from build123d import *

# Parameters (mm, degrees)
BOSS_EXTRUDE1_DEPTH  = 8.6
CHAMFER1_SIZE        = 1.414
CHAMFER1_EDGE_2_SIZE = 1.414
CHAMFER1_EDGE_3_SIZE = 1.414
CHAMFER1_EDGE_4_SIZE = 1.414
CHAMFER1_EDGE_5_SIZE = 1.414
CHAMFER1_EDGE_6_SIZE = 1.414
FILLET2_R            = 0.25
SKETCH6_R            = 1.5
CUT_EXTRUDE1_DEPTH   = 28
BOSS_EXTRUDE2_DEPTH  = 2.1
SKETCH9_R            = 2.75
CUT_EXTRUDE2_DEPTH   = 4.2
CHAMFER3_SIZE        = 0.75


with BuildPart() as part:
    # Sketch1 → Revolve1 (revolve)
    with BuildSketch(Plane.XY, mode=Mode.PRIVATE) as revolve1_sk:
        Polygon((0, 0), (6, 0), (6, 5.75), (4.875, 5.75), (4.875, 6.5), (7.75, 8), (7.75, 38.4), (8.7, 38.4), (8.7, 39.4), (0, 39.4), align=None)
    revolve(revolve1_sk.sketch.rotate(Axis((0, 39.4, 0), (0, -1, 0)), 180), axis=Axis((0, 39.4, 0), (0, -1, 0)))

    # Sketch3 → Boss-Extrude1 (add)
    with BuildSketch(Plane(origin=(0, 39.4, 0), x_dir=(1, 0, 0), z_dir=(0, 1, 0))):
        Polygon((0, 9.814954576), (-8.5, 4.907477288), (-8.5, -4.907477288), (0, -9.814954576), (8.5, -4.907477288), (8.5, 4.907477288), align=None)
    extrude(amount=BOSS_EXTRUDE1_DEPTH)

    # Chamfer1
    chamfer1_edges = [part.edges().sort_by_distance(p)[0] for p in [
        (8.5, 43.7, -4.907477288),
    ]]
    chamfer(chamfer1_edges, length=CHAMFER1_SIZE)

    # Chamfer1 edge 2
    chamfer1_edge_2_edges = [part.edges().sort_by_distance(p)[0] for p in [
        (0, 43.7, -9.814954576),
    ]]
    chamfer(chamfer1_edge_2_edges, length=CHAMFER1_EDGE_2_SIZE)

    # Chamfer1 edge 3
    chamfer1_edge_3_edges = [part.edges().sort_by_distance(p)[0] for p in [
        (-8.5, 43.7, -4.907477288),
    ]]
    chamfer(chamfer1_edge_3_edges, length=CHAMFER1_EDGE_3_SIZE)

    # Chamfer1 edge 4
    chamfer1_edge_4_edges = [part.edges().sort_by_distance(p)[0] for p in [
        (-8.5, 43.7, 4.907477288),
    ]]
    chamfer(chamfer1_edge_4_edges, length=CHAMFER1_EDGE_4_SIZE)

    # Chamfer1 edge 5
    chamfer1_edge_5_edges = [part.edges().sort_by_distance(p)[0] for p in [
        (0, 43.7, 9.814954576),
    ]]
    chamfer(chamfer1_edge_5_edges, length=CHAMFER1_EDGE_5_SIZE)

    # Chamfer1 edge 6
    chamfer1_edge_6_edges = [part.edges().sort_by_distance(p)[0] for p in [
        (8.5, 43.7, 4.907477288),
    ]]
    chamfer(chamfer1_edge_6_edges, length=CHAMFER1_EDGE_6_SIZE)

    # Sketch5 → Revolve2 (revolve)
    with BuildSketch(Plane.XY, mode=Mode.PRIVATE) as revolve2_sk:
        Polygon((7.75, 28.801965379), (10.5, 28.801965379), (10.5, 26.801965379), (8.7, 26.801965379), (8.7, 23.801965379), (7.75, 23.801965379), align=None)
    revolve(revolve2_sk.sketch.rotate(Axis((0, 0, 0), (0, 1, 0)), 180), axis=Axis((0, 0, 0), (0, 1, 0)))

    # Fillet2
    fillet2_edges = [part.edges().sort_by_distance(p)[0] for p in [
        (10.5, 28.801965379, 0),
        (10.5, 26.801965379, 0),
        (8.7, 23.801965379, 0),
    ]]
    fillet(fillet2_edges, radius=FILLET2_R)

    # Sketch6 → Cut-Extrude1 (cut)
    with BuildSketch(Plane.XZ):
        Circle(SKETCH6_R)
    extrude(amount=-CUT_EXTRUDE1_DEPTH, mode=Mode.SUBTRACT)

    # Sketch7 → Boss-Extrude2 (add, symmetric)
    with BuildSketch(Plane.XY):
        with BuildLine():
            Line((4.5, 54.25), (4.5, 48))
            Line((4.5, 48), (-4.5, 48))
            Line((-4.5, 48), (-4.5, 54.25))
            ThreePointArc((-4.5, 54.25), (0, 58.75), (4.5, 54.25))
        make_face()
    extrude(amount=BOSS_EXTRUDE2_DEPTH, both=True)

    # Sketch8 → Cut-Revolve1 (revolve, cut)
    with BuildSketch(Plane.XY):
        with BuildLine():
            Line((0, 57.15), (0, 51.35))
            ThreePointArc((0, 51.35), (2.9, 54.25), (0, 57.15))
        make_face()
    revolve(axis=Axis((0, 48, 0), (0, 1, 0)), mode=Mode.SUBTRACT)

    # Sketch10 → Cut-Revolve2 (revolve, cut)
    with BuildSketch(Plane.XY, mode=Mode.PRIVATE) as cut_revolve2_sk:
        Polygon((7, 48), (8.5, 46.6), (10.124681139, 45.083630937), (10.124681139, 47.819402207), (7, 50.73577127), align=None)
    revolve(cut_revolve2_sk.sketch.rotate(Axis((0, 0, 0), (0, 1, 0)), 90), axis=Axis((0, 0, 0), (0, 1, 0)), mode=Mode.SUBTRACT)

    # Sketch9 → Cut-Extrude2 (cut)
    with BuildSketch(Plane.XY.offset(2.1)):
        with Locations((0, 54.25)):
            Circle(SKETCH9_R)
    extrude(amount=-CUT_EXTRUDE2_DEPTH, mode=Mode.SUBTRACT)

    # Chamfer3
    chamfer3_edges = [part.edges().sort_by_distance(p)[0] for p in [
        (6, 0, 0),
    ]]
    chamfer(chamfer3_edges, length=CHAMFER3_SIZE)


solid = part.part
Input: part model. Units: mm. Frame: model coordinates. A direction names the side the tool comes from. Give positions to 0.01 mm unless a question says otherwise; leave off trailing zeros. Write each loop counter-clockwise with the first axis right and the second up, starting at its lowest first coordinate (ties: lowest second). Pieces come first, ordered by that corner, then holes. Notation, with made-up numbers: M 44,16 L 56,16 A22 ccw 56,42 Z; hole C 69.5,-37.75 d3. An arc over 180 degrees is marked long. Write item = value, one per line. Start each with the question number.
1) Cut plane A-A on y = 50. Return the cut outline in (x, z).
2) First-contact query: pin 1 Ø8 at (y, z) = (46.5, -4) entering from -X; pin 2 Ø2 at (y, z) = (50, -0.5) entering from +X; pin 3 Ø2 at (x, y) = (-5, 28.5) entering from +Z. Flat tips, straight axial feed; report the tip coordinate or a pass-through.
3) Cut plane B-B on y = 30.5. Return the cut outline in (x, z), then the cut area to 3 significant figures.
4) Material intervals for line 1 along Z through (x, y) = (0, 13.25); line 2 along X through (y, z) = (54.25, -1.7); line 3 along Y through (x, z) = (0, -1.75), sorted ascending. Write a range as [from, to].
5) Reachability of faces 1 (the flat face through (7.896, 42.67, -4.539)), 2 (the cylindrical face through (1.009, 16.012, -7.684)), 3 (the cylindrical face through (1.886, 38.907, 8.493)) from +Z, -Z, +X, -X, +Y, -Y: full face, straight path, thin tool, end or side. Return the list, or none.
6) Draft query along Y for faces 4 (the flat face through (8, 39.4, 4)), 5 (the flat face through (4.208, 42.95, 7.386)), 6 (the flat face through (-4, 23.802, -7)), 7 (the cylindrical face through (-0.358, 56.977, 1.519)). Return one class per face: +Y half, -Y half, draft (parallel to the pull), parting line (faces both ways), or undercut.
Solved:
q1.outline = M -4.5,-2.1 L 4.5,-2.1 L 4.5,2.1 L -4.5,2.1 Z
q2.pin_1 = -8.5
q2.pin_2 = 4.5
q2.pin_3 = 9.71
q3.outline = C 0,0 d15.5
q3.area = 189 mm2
q4.line_1 = [-7.75, -1.5], [1.5, 7.75]
q4.line_2 = [-4.5, -2.75], [2.75, 4.5]
q4.line_3 = [0, 51.5], [57, 58.75]
q5.face_1 = -Z, +X, +Y
q5.face_2 = -Y
q5.face_3 = none
q6.face_4 = undercut
q6.face_5 = draft
q6.face_6 = -Y half
q6.face_7 = undercut
